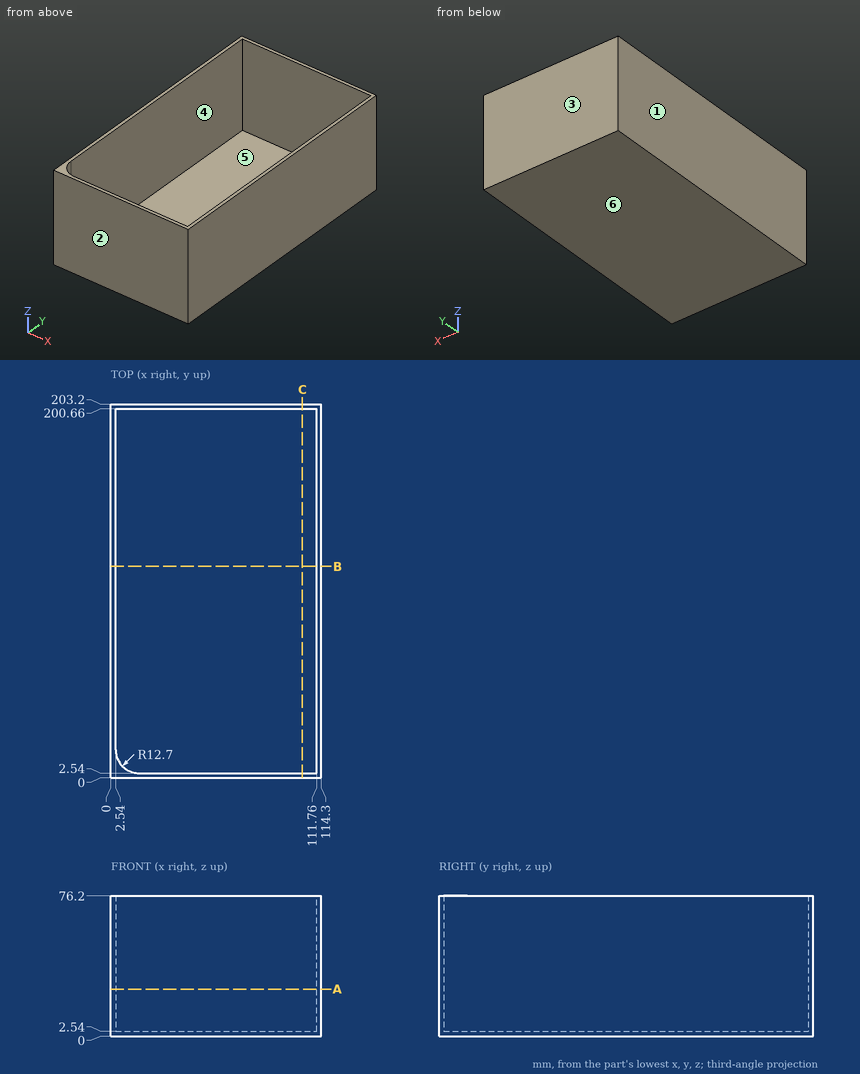
Answer from the drawing. Dimensions are ordinates in mm from the lowest x, y and z of the part. A direction names the side the tool comes from. Give positions to 0.01 mm unless a question says otherwise; leave off trailing zeros. Write each loop counter-clockwise with the first axis right and the second up, starting at its lowest first coordinate (ties: lowest second). Pieces come first, ordered by that corner, then holes. Notation, with made-up numbers: (36.25, 41.5) -> (80.25, 41.5) arc R30 ccw to (80.25, 64.5) -> close; hole circle Ø11 at (84.5, 52.25). An arc over 180 degrees is marked (long way). One line per question, with ' | ' between items. Start each with the question number.
1. Section C-C (x = 104) is taken. Determine the outline of the cut face in (y, z).
2. Given pin 1 Ø2 at (x, y) = (32.5, 174) entering from +Z, flat-ended and moving along its own axis, determine where the tip first touches the part or whether it passes through.
3. Section B-B (y = 115) is taken. Determine the outline of the cut face in (x, z), plus the area to 3 significant figures.
4. Find the intervals of material crossed by probe 1 along Y at (x, z) = (80, 41); probe 2 along X at (y, z) = (73.5, 41.5); probe 3 along Z at (x, y) = (46, 115.5), in increasing order.
5. Section A-A (z = 25.5) is taken. Determine the outline of the cut face in (x, y), plus the area to 3 significant figures.
6. For the marked faces 5 and 6, determine the directions among +Z, -Z, +X, -X, +Y, -Y from which every point of the face is accessible in a straight line to the end or side of a thin tool.
7. For a pull along Y with two mould halves and no side action, classify the marked faces 1, 2, 3 and 4 as pulls with the +Y half, pulls with the -Y half, needs draft (parallel to the pull), parting line crosses it, or undercut.
Response values:
1) outline: (0, 0) -> (203.2, 0) -> (203.2, 76.2) -> (200.66, 76.2) -> (200.66, 2.54) -> (2.54, 2.54) -> (2.54, 76.2) -> (0, 76.2) -> close
2) pin 1: z = 2.54
3) outline: (0, 0) -> (114.3, 0) -> (114.3, 76.2) -> (111.76, 76.2) -> (111.76, 2.54) -> (2.54, 2.54) -> (2.54, 76.2) -> (0, 76.2) -> close | area: 665 mm2
4) probe 1: 0 to 2.54, 200.66 to 203.2 | probe 2: 0 to 2.54, 111.76 to 114.3 | probe 3: 0 to 2.54
5) outline: (0, 0) -> (114.3, 0) -> (114.3, 203.2) -> (0, 203.2) -> close; hole (2.54, 15.24) arc R12.7 ccw to (15.24, 2.54) -> (111.76, 2.54) -> (111.76, 200.66) -> (2.54, 200.66) -> close | area: 1,620 mm2
6) face 5: +Z | face 6: -Z, +X, -X, +Y, -Y
7) face 1: needs draft | face 2: pulls with the -Y half | face 3: pulls with the +Y half | face 4: undercut
